from build123d import *

# Parameters (mm, degrees)
SKETCH1_W           = 50
SKETCH1_H           = 50
BOSS_EXTRUDE1_DEPTH = 30
SKETCH2_R           = 13.5
CUT_EXTRUDE1_DEPTH  = 26
BOSS_EXTRUDE2_DEPTH = 20
BOSS_EXTRUDE3_DEPTH = 20
CUT_EXTRUDE2_DEPTH  = 20
CUT_EXTRUDE3_DEPTH  = 20
CHAMFER1_SIZE       = 2
SKETCH4_R           = 3.1
CUT_EXTRUDE4_DEPTH  = 2.5
CHAMFER2_SIZE       = 1
CHAMFER3_SIZE       = 2.5


with BuildPart() as part:
    # Sketch1 → Boss-Extrude1 (new body)
    with BuildSketch(Plane(origin=(0, 0, 0), x_dir=(1, 0, 0), z_dir=(0, 1, 0))):
        with Locations((25, 25)):
            Rectangle(SKETCH1_W, SKETCH1_H)
    extrude(amount=BOSS_EXTRUDE1_DEPTH)

    # Sketch2 → Cut-Extrude1 (cut)
    with BuildSketch(Plane(origin=(0, 30, 0), x_dir=(1, 0, 0), z_dir=(0, 1, 0))):
        with Locations(Location((25, 25, 0), (0, 0, 270))):
            Circle(SKETCH2_R)
    extrude(amount=-CUT_EXTRUDE1_DEPTH, mode=Mode.SUBTRACT)

    # Sketch3 → Boss-Extrude2 (add)
    with BuildSketch(Plane(origin=(0, 0, 0), x_dir=(1, 0, 0), z_dir=(0, 1, 0))):
        Polygon((50, 33.556624327), (52.5, 35), (52.5, 15), (50, 16.443375673), align=None)
    extrude(amount=BOSS_EXTRUDE2_DEPTH)

    # Sketch3<3> → Boss-Extrude3 (add)
    with BuildSketch(Plane(origin=(0, 0, 0), x_dir=(1, 0, 0), z_dir=(0, 1, 0))):
        Polygon((16.443375673, 50), (15, 52.5), (35, 52.5), (33.556624327, 50), align=None)
    extrude(amount=BOSS_EXTRUDE3_DEPTH)

    # Sketch3<4> → Cut-Extrude2 (cut)
    with BuildSketch(Plane(origin=(0, 0, 0), x_dir=(1, 0, 0), z_dir=(0, 1, 0))):
        Polygon((0, 33.556624327), (2.5, 35), (2.5, 15), (0, 16.443375673), align=None)
    extrude(amount=CUT_EXTRUDE2_DEPTH, mode=Mode.SUBTRACT)

    # Sketch3<5> → Cut-Extrude3 (cut)
    with BuildSketch(Plane(origin=(0, 0, 0), x_dir=(1, 0, 0), z_dir=(0, 1, 0))):
        Polygon((16.443375673, 0), (15, 2.5), (35, 2.5), (33.556624327, 0), align=None)
    extrude(amount=CUT_EXTRUDE3_DEPTH, mode=Mode.SUBTRACT)

    # Chamfer1
    chamfer1_edges = [part.edges().sort_by_distance(p)[0] for p in [
        (50, 30, -25),
        (25, 30, -38.5),
        (25, 30, -50),
        (0, 30, -25),
        (25, 30, 0),
    ]]
    chamfer(chamfer1_edges, length=CHAMFER1_SIZE)

    # Sketch4 → Cut-Extrude4 (cut)
    with BuildSketch(Plane(origin=(0, 0, 0), x_dir=(1, 0, 0), z_dir=(0, 1, 0))):
        with Locations(Location((12.5, 37.5, 0), (0, 0, 270))):
            Circle(SKETCH4_R)
        with Locations(Location((37.5, 37.5, 0), (0, 0, 270))):
            Circle(SKETCH4_R)
        with Locations(Location((37.5, 12.5, 0), (0, 0, 270))):
            Circle(SKETCH4_R)
        with Locations(Location((12.5, 12.5, 0), (0, 0, 270))):
            Circle(SKETCH4_R)
    extrude(amount=CUT_EXTRUDE4_DEPTH, mode=Mode.SUBTRACT)

    # Chamfer2
    chamfer2_edges = [part.edges().sort_by_distance(p)[0] for p in [
        (12.5, 2.5, -40.6),
        (12.5, 2.5, -15.6),
        (37.5, 2.5, -15.6),
        (37.5, 2.5, -40.6),
    ]]
    chamfer(chamfer2_edges, length=CHAMFER2_SIZE)

    # Chamfer3
    chamfer3_edges = [part.edges().sort_by_distance(p)[0] for p in [
        (0, 20, -25),
        (25, 20, 0),
    ]]
    chamfer(chamfer3_edges, length=CHAMFER3_SIZE - 0.0001)  # a hair under: the kernel refuses the full size


solid = part.part
Verification items for the finished model (mm, model axes). A direction names the side the tool comes from. Give positions to 0.01 mm unless a question says otherwise; leave off trailing zeros. Write each loop counter-clockwise with the first axis right and the second up, starting at its lowest first coordinate (ties: lowest second). Pieces come first, ordered by that corner, then holes.
(1) Material ranges on line 1 (X direction, y = 0.45, z = -37.5); line 2 (Y direction, x = 14, z = -37.5); line 3 (X direction, y = 21.5, z = -49), recorded low to high.
(2) Cross-section at A-A (y = 18.5). Enter the section's corners in (x, z), plus the area to 3 significant figures.
(3) Cross-section at C-C (x = 5). Enter the section's corners in (y, z), plus the area to 3 significant figures.
(4) Mould release check, pull along Z, two halves, no side actions. Record for faces 4 (the face through (1.27, 11.09, -15.71)), 5 (the face through (51.27, 9.86, -15.71)), 6 (the face through (15.732, 11.092, -1.233)), 7 (the face through (0, 23, -25)): +Z half, -Z half, draft (parallel to the pull), parting line (faces both ways), or undercut.
(5) Cross-section at D-D (z = -45). Enter the section's corners in (x, y), plus the area to 3 significant figures.
(6) Access from +Z, -Z, +X, -X, +Y, -Y to the whole of each face (thin tool, end or side, straight path). Record for faces 1 (the face through (19.83, 16.17, -12.53)), 2 (the face through (13.431, 0.74, -34.543)), 3 (the face through (51.232, 9.86, -34.268)).
(7) Gauge pin test, flat ends, axial feed: pin 1 (10 mm diameter, centred on x = 9, y = 16.5, fed in from -Z); pin 2 (10 mm diameter, centred on x = 14.5, y = 3, fed in from +Z); pin 3 (0.8 mm diameter, centred on x = 51.5, z = -21.5, fed in from +Y); pin 4 (4.5 mm diameter, centred on x = 12, z = -12.5, fed in from -Y). Record the tip position at first contact, or that the pin passes through.
Worked out:
1. line 1: x = 0 to 9.4, 15.6 to 34.4, 40.6 to 50
1. line 2: y = 2.5 to 30
1. line 3: x = 0 to 50
2. outline: (0, -50) - (16.44, -50) - (15, -52.5) - (35, -52.5) - (33.56, -50) - (50, -50) - (50, -33.56) - (52.5, -35) - (52.5, -15) - (50, -16.44) - (50, 0) - (33.56, 0) - (35, -2.5) - (15, -2.5) - (16.44, 0) - (0, 0) - (0, -16.44) - (2.5, -15) - (2.5, -35) - (0, -33.56) - close; hole circle Ø27 at (25, -25)
2. area: 1,930 mm2
3. outline: (0, -50) - (28, -50) - (30, -48) - (30, -2) - (28, 0) - (0, 0) - close
3. area: 1,500 mm2
4. face 4: undercut
4. face 5: +Z half
4. face 6: undercut
4. face 7: draft
5. outline: (0, 0) - (50, 0) - (50, 28) - (48, 30) - (2, 30) - (0, 28) - close
5. area: 1,500 mm2
6. face 1: +Y
6. face 2: -Y
6. face 3: -Z, +Y, -Y
7. pin 1: stops at z = -50
7. pin 2: stops at z = 0
7. pin 3: stops at y = 20
7. pin 4: stops at y = 1.85
